```python
from build123d import *

# Parameters (mm, degrees)
F0_W     = 50.8
F0_H     = 50.8
F1_DEPTH = 50.8


with BuildPart() as f1:
    # F0 (on Front) → F1 (new body)
    with BuildSketch(Plane.XZ):
        with Locations((-25.4, 25.4)):
            Rectangle(F0_W, F0_H)
    extrude(amount=F1_DEPTH)

    # F2 (on face) → F3 (revolve, cut)
    with BuildSketch(Plane.YZ):
        with BuildLine():
            Line((-19.3643093263, 19.3643093263), (-31.4356906737, 31.4356906737))
            ThreePointArc((-31.4356906737, 31.4356906737), (-31.4356906737, 19.3643093263), (-19.3643093263, 19.3643093263))
        make_face()
    revolve(axis=Axis((0, -25.4, 25.4), (0, 0.7071067812, -0.7071067812)), mode=Mode.SUBTRACT)

    # F4 (on face) → F5 (revolve, cut)
    with BuildSketch(Plane.XY.offset(50.8)):
        with BuildLine():
            ThreePointArc((-28.7345517881, -15.7154482119), (-32.6545119926, -9.8488131804), (-39.5746798487, -11.2253201513))
            Line((-39.5746798487, -11.2253201513), (-30.5944237276, -20.2055762724))
            ThreePointArc((-30.5944237276, -20.2055762724), (-29.2179167567, -18.1454880074), (-28.7345517881, -15.7154482119))
        make_face()
        with BuildLine():
            ThreePointArc((-9.3654482119, -35.0845517881), (-13.2854084164, -29.2179167567), (-20.2055762724, -30.5944237276))
            Line((-20.2055762724, -30.5944237276), (-11.2253201513, -39.5746798487))
            ThreePointArc((-11.2253201513, -39.5746798487), (-9.8488131804, -37.5145915836), (-9.3654482119, -35.0845517881))
        make_face()
    revolve(axis=Axis((-25.4, -25.4, 50.8), (0.7071067812, -0.7071067812, 0)), mode=Mode.SUBTRACT)


solid = f1.part
```
Geometry: final body of the model. Coordinates: model frame, mm. Coordinates: 2 decimals unless noted, no trailing zeros. Order: outer loops, then holes, each group sorted by start corner. A loop starts at its lowest first (then second) coordinate and runs counter-clockwise, first axis right, second up. Notation, with made-up numbers: (66.5, -24) -> (80.5, -24) arc R16 ccw to (80.5, -15) -> close; hole circle Ø1 at (-32, 57). An arc over 180 degrees is marked (long way). Use CSV: the item, a comma, the result in double quotes.
1) Section A-A on x = -14. Output: boundary loops of the cut face in (y, z).
Findings:
outline,"(-50.8, 0) -> (0, 0) -> (0, 50.8) -> (-28.97, 50.8) arc R6.11 cw to (-41.2, 50.8) -> (-50.8, 50.8) -> close"
2) Section B-B on z = 47.5. Output: boundary loops of the cut face in (x, y), then the cut area to 3 significant figures.
Findings:
outline,"(-50.8, -50.8) -> (0, -50.8) -> (0, 0) -> (-50.8, 0) -> close; hole circle Ø10.85 at (-35.08, -15.72); hole circle Ø10.85 at (-15.72, -35.08)"
area,"2,400 mm^2"
3) Section D-D on y = -18.5. Output: boundary loops of the cut face in (x, z).
Findings:
outline,"(-50.8, 0) -> (0, 0) -> (0, 20.38) arc R5.02 cw to (0, 30.42) -> (0, 50.8) -> (-29.38, 50.8) arc R5.71 cw to (-40.79, 50.8) -> (-50.8, 50.8) -> close"
4) Line query: line 1 (Y direction, x = -17.5, z = 47.5); line 2 (Z direction, x = -37, y = -13); line 3 (Z direction, x = -40.5, y = -15.5). Output: solid intervals per line, ascending.
Findings:
line 1,"y = -50.8 to -40.21, -29.96 to 0"
line 2,"z = 0 to 45.39"
line 3,"z = 0 to 47.49"
5) Section C-C on z = 22.5. Output: boundary loops of the cut face in (x, y), then the cut area to 3 significant figures.
Findings:
outline,"(-50.8, -50.8) -> (0, -50.8) -> (0, -33.43) arc R8.03 cw to (0, -17.37) -> (0, 0) -> (-50.8, 0) -> close"
area,"2,480 mm^2"
